The listing builds one solid part. Answer for the finished solid, in the listing's coordinates (mm). A direction names the side the tool comes from. Round coordinates to 2 decimals unless told otherwise and drop trailing zeros. Loops run counter-clockwise (first coordinate to the right, second up) from the corner with the lowest first, then second, coordinate; pieces in that order, holes last. Notation, with made-up numbers: (65.5, -7) - (111.5, -7) arc R26 cw to (111.5, 28) - close; hole circle Ø8 at (57, 52). An arc over 180 degrees is marked (long way). Write item = value, one per line. Start each with the question number.
1) Section D-D, the plane y = -5 is taken. Determine the outline of the cut face in (x, z).
2) Straight lines are drawn through the part: line 1 along X through (y, z) = (-4.75, 6.5); line 2 along Z through (x, y) = (21.5, 0); line 3 along Y through (x, z) = (64, 3.5). For each, find the intervals that lie inside material, in ascending order.
3) Section C-C, the plane x = 103.5 is taken. Determine the outline of the cut face in (y, z) (1 decimal), and give its area (3 significant figures).
4) Section A-A, the plane z = 0 is taken. Determine the outline of the cut face in (x, y), and give its area (3 significant figures).
5) A tool of negligible diameter and unlimited length cuts with its end or side. For faces 1 (the flat face through (101, 2.388, 12)), 2 (the cylindrical face through (133.17, 6.2, -1.38)), 3 (the flat face through (101, -2.388, 12)), from which of +Z, -Z, +X, -X, +Y, -Y can it reach the whole face along a straight path? Write none if from no direction.
6) Given pin 1 Ø2 at (y, z) = (-3.5, -8) entering from +X; pin 2 Ø6 at (x, y) = (77, 4.5) entering from +Z; pin 3 Ø5 at (x, z) = (91, -6) entering from -Y, each flat-ended and moving along its own axis, determine where each tip first touches the part or whether it passes through.
from build123d import *

# Parameters (mm, degrees)
F3_DEPTH = 39.65
F4_DEPTH = 12.7
F5_DEPTH = 12.7


with BuildPart() as f1:
    # F0 (on Front) → F1 (revolve)
    with BuildSketch(Plane.XZ):
        Polygon((0, 6.35), (0, 0), (133.35, 0), (133.35, 6.35), (120.65, 6.35), (120.65, 11.1125), (80.9773877263, 11.1125), (80.9773877263, 6.35), align=None)
    revolve(axis=Axis((66.675, 0, 0), (1, 0, 0)))

    # F2 (on face) → F3 (join)
    with BuildSketch(Plane.YZ.offset(120.65)):
        with BuildLine():
            Line((-2.3876, 13.1389729793), (-2.3876, 10.8529729793))
            ThreePointArc((-2.3876, 10.8529729793), (0, 11.1125), (2.3876, 10.8529729793))
            Line((2.3876, 10.8529729793), (2.3876, 13.1389729793))
            Line((2.3876, 13.1389729793), (-2.3876, 13.1389729793))
        make_face()
    extrude(amount=-F3_DEPTH)

    # F4 (add): a face of the model
    f4_faces = [f1.faces().sort_by_distance(p)[0] for p in [
        (133.35, 0, 0),
    ]]
    extrude(f4_faces, amount=F4_DEPTH)

    # F5 (cut): a face of the model
    f5_faces = [f1.faces().sort_by_distance(p)[0] for p in [
        (0, 0, 0),
    ]]
    extrude(f5_faces, amount=-F5_DEPTH, mode=Mode.SUBTRACT)


solid = f1.part
Geometry check:
q1.outline = (12.7, -3.91) - (80.98, -3.91) - (80.98, -9.92) - (120.65, -9.92) - (120.65, -3.91) - (146.05, -3.91) - (146.05, 3.91) - (120.65, 3.91) - (120.65, 9.92) - (80.98, 9.92) - (80.98, 3.91) - (12.7, 3.91) - close
q2.line_1 = 80.98 to 120.65
q2.line_2 = -6.35 to 6.35
q2.line_3 = -5.3 to 5.3
q3.outline = (-2.4, 10.9) arc R11.1 ccw (long way) to (2.4, 10.9) - (2.4, 13.1) - (-2.4, 13.1) - close
q3.area = 398 mm2
q4.outline = (12.7, -6.35) - (80.98, -6.35) - (80.98, -11.11) - (120.65, -11.11) - (120.65, -6.35) - (146.05, -6.35) - (146.05, 6.35) - (120.65, 6.35) - (120.65, 11.11) - (80.98, 11.11) - (80.98, 6.35) - (12.7, 6.35) - close
q4.area = 2,070 mm2
q5.face_1 = +Z, +X, -X, +Y
q5.face_2 = +X
q5.face_3 = +Z, +X, -X, -Y
q6.pin_1 = 120.65
q6.pin_2 = 6.17
q6.pin_3 = -10.55
